Design review of the part built by this model. Coordinates are the model's own, in mm. A direction names the side the tool comes from. Coordinates: 2 decimals unless noted, no trailing zeros. Write each loop counter-clockwise with the first axis right and the second up, starting at its lowest first coordinate (ties: lowest second). Pieces come first, ordered by that corner, then holes. Notation, with made-up numbers: (-34, -32) - (20, -32) arc R20 ccw to (20, 5) - close; hole circle Ø5 at (62.5, -29.75). An arc over 180 degrees is marked (long way). One line per item, written item: value.
from build123d import *

# Parameters (mm, degrees)
ESQUISSE1_W             = 77
ESQUISSE1_H             = 17
BOSS_EXTRU_1_DEPTH      = 2
ESQUISSE2_W             = 60
ESQUISSE2_H             = 9
ESQUISSE2_W_2           = 58
ESQUISSE2_H_2           = 7
ENL_V_MAT_EXTRU_1_DEPTH = 1
ESQUISSE3_W             = 8.5
ESQUISSE3_H             = 6
BOSS_EXTRU_2_DEPTH      = 3.5
ESQUISSE4_R             = 1.75
ESQUISSE4_R_2           = 0.75
ENL_V_MAT_EXTRU_2_DEPTH = 3
ESQUISSE5_W             = 7
ESQUISSE5_H             = 2.5
ESQUISSE5_W_2           = 2.5
ESQUISSE5_H_2           = 5.5
ESQUISSE5_W_3           = 4
ESQUISSE5_H_3           = 3
BOSS_EXTRU_3_DEPTH      = 1.5


with BuildPart() as part:
    # Esquisse1 → Boss.-Extru.1 (new body)
    with BuildSketch(Plane(origin=(0, 0, 0), x_dir=(1, 0, 0), z_dir=(0, 1, 0))):
        with Locations((38.5, 8.5)):
            Rectangle(ESQUISSE1_W, ESQUISSE1_H)
    extrude(amount=BOSS_EXTRU_1_DEPTH)

    # Esquisse2 → Enlèv. mat.-Extru.1 (cut)
    with BuildSketch(Plane(origin=(0, 2, 0), x_dir=(1, 0, 0), z_dir=(0, 1, 0))):
        with Locations((38.5, 5.5)):
            Rectangle(ESQUISSE2_W, ESQUISSE2_H)
        with Locations((38.5, 5.5)):
            Rectangle(ESQUISSE2_W_2, ESQUISSE2_H_2, mode=Mode.SUBTRACT)
    extrude(amount=-ENL_V_MAT_EXTRU_1_DEPTH, mode=Mode.SUBTRACT)

    # Esquisse3 → Boss.-Extru.2 (add)
    with BuildSketch(Plane(origin=(0, 2, 0), x_dir=(1, 0, 0), z_dir=(0, 1, 0))):
        with Locations((4.25, 3)):
            Rectangle(ESQUISSE3_W, ESQUISSE3_H)
    extrude(amount=BOSS_EXTRU_2_DEPTH)

    # Esquisse4 → Enlèv. mat.-Extru.2 (cut, through all)
    with BuildSketch(Plane(origin=(0, 2, 0), x_dir=(1, 0, 0), z_dir=(0, 1, 0))):
        with Locations((74, 11)):
            Circle(ESQUISSE4_R)
        with Locations((49, 12)):
            Circle(ESQUISSE4_R_2)
        with Locations((3, 11)):
            Circle(ESQUISSE4_R)
        with Locations((28, 12)):
            Circle(ESQUISSE4_R_2)
    extrude(amount=-ENL_V_MAT_EXTRU_2_DEPTH, mode=Mode.SUBTRACT)

    # Esquisse5 → Boss.-Extru.3 (add)
    with BuildSketch(Plane.XZ):
        with Locations((4, -1.75)):
            Rectangle(ESQUISSE5_W, ESQUISSE5_H)
        with Locations((8.25, -5.85)):
            Rectangle(ESQUISSE5_W_2, ESQUISSE5_H_2)
        with Locations((15, -10.5)):
            Rectangle(ESQUISSE5_W_3, ESQUISSE5_H_3)
        with Locations((13.5, -2)):
            Rectangle(ESQUISSE5_W_3, ESQUISSE5_H_3)
        with Locations((68.75, -5.85)):
            Rectangle(ESQUISSE5_W_2, ESQUISSE5_H_2)
        with Locations((62, -10.5)):
            Rectangle(ESQUISSE5_W_3, ESQUISSE5_H_3)
        with Locations((63.5, -2)):
            Rectangle(ESQUISSE5_W_3, ESQUISSE5_H_3)
    extrude(amount=BOSS_EXTRU_3_DEPTH)


solid = part.part
1. For faces 1 (the face through (7.5, -1, -2)), 2 (the face through (63, -1, -3.5)), 3 (the face through (62, -1, -12)), 4 (the face through (70, -1, -6)), list the 3-axis set-ups (+Z, -Z, +X, -X, +Y, -Y) from which the entire face can be reached by the end or side of a thin tool; tool diameter is ignored.
Answer block:
face 1: +Z, -Y
face 2: -Y
face 3: -Z, +X, -X, -Y
face 4: +Z, -Z, +X, -Y
2. Insertion check: pin 1 Ø0.8 at (y, z) = (-0.5, -11) entering from +X; pin 2 Ø0.8 at (x, y) = (62.5, -1) entering from +Z; pin 3 Ø1.2 at (x, y) = (68.5, -1) entering from +Z. Each pin has a flat end and moves straight along its axis. Give the tip position at first contact, or say it passes through.
Answer block:
pin 1: stops at x = 64
pin 2: stops at z = -0.5
pin 3: stops at z = -3.1
3. Wall thickness on line 1 along X through (y, z) = (0.55, -11); line 2 along X through (y, z) = (1.5, -5.5); line 3 along Z through (x, y) = (36, 1.75): over which ranges is each line inside the solid? List them lowest first.
Answer block:
line 1: x = 0 to 1.25, 4.75 to 72.25, 75.75 to 77
line 2: x = 0 to 8.5, 9.5 to 67.5, 68.5 to 77
line 3: z = -17 to -10, -9 to -2, -1 to 0
4. Consider section D-D, the plane x = 3. Write out the cut boundary in (y, z), then the cut area to 4 significant figures.
Answer block:
outline: (-1.5, -3) - (0, -3) - (0, -9.25) - (2, -9.25) - (2, -6) - (5.5, -6) - (5.5, 0) - (0, 0) - (0, -0.5) - (-1.5, -0.5) - close; (0, -17) - (2, -17) - (2, -12.75) - (0, -12.75) - close
area: 51.75 mm^2
5. Consider section B-B, the plane z = -7.5. Write out the cut boundary in (x, y).
Answer block:
outline: (0, 0) - (7, 0) - (7, -1.5) - (9.5, -1.5) - (9.5, 0) - (67.5, 0) - (67.5, -1.5) - (70, -1.5) - (70, 0) - (77, 0) - (77, 2) - (68.5, 2) - (68.5, 1) - (67.5, 1) - (67.5, 2) - (9.5, 2) - (9.5, 1) - (8.5, 1) - (8.5, 2) - (0, 2) - close
6. Consider section C-C, the plane x = 14.5. Write out the cut boundary in (y, z).
Answer block:
outline: (-1.5, -12) - (0, -12) - (0, -17) - (2, -17) - (2, -10) - (1, -10) - (1, -9) - (2, -9) - (2, -2) - (1, -2) - (1, -1) - (2, -1) - (2, 0) - (0, 0) - (0, -0.5) - (-1.5, -0.5) - (-1.5, -3.5) - (0, -3.5) - (0, -9) - (-1.5, -9) - close
7. Consider section A-A, the plane x = 74. Write out the cut boundary in (y, z).
Answer block:
outline: (0, -17) - (2, -17) - (2, -12.75) - (0, -12.75) - close; (0, -9.25) - (2, -9.25) - (2, 0) - (0, 0) - close
